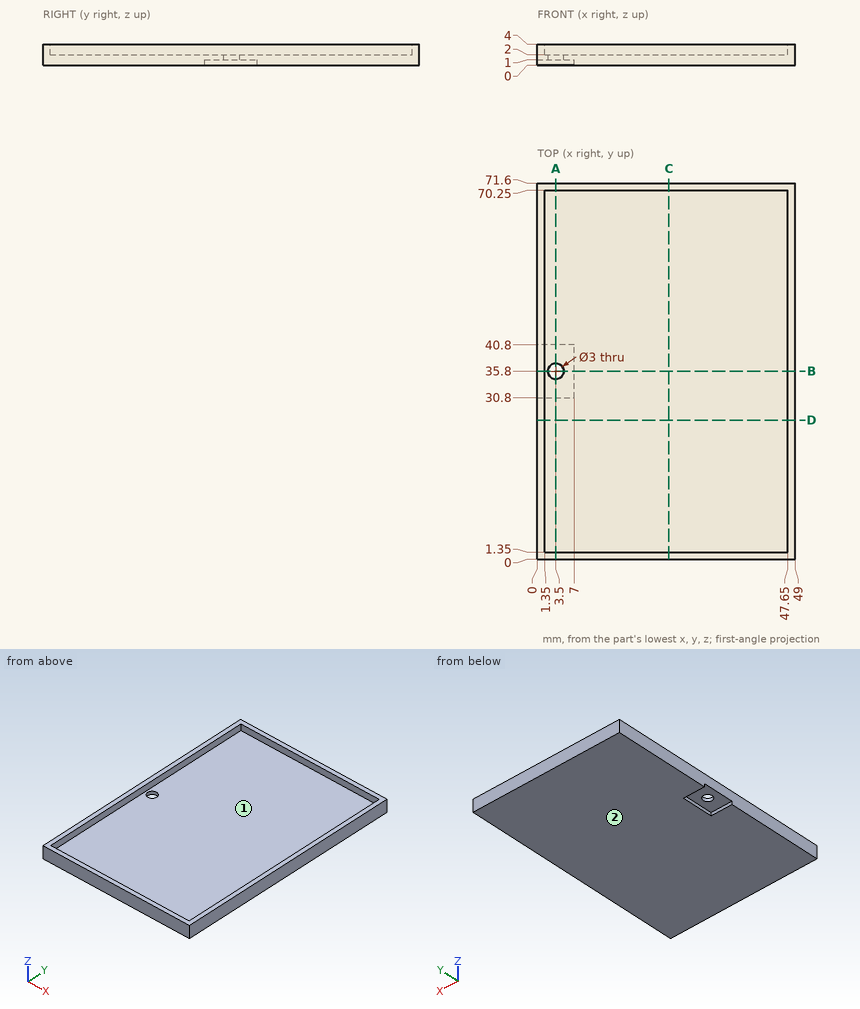
Print and shaded views of the part. All mm, measured from the part's lowest x, y and z. Round coordinates to 2 decimals unless told otherwise and drop trailing zeros. Write each loop counter-clockwise with the first axis right and the second up, starting at its lowest first coordinate (ties: lowest second). Pieces come first, ordered by that corner, then holes. Notation, with made-up numbers: M 12,4 L 52,4 A14 ccw 52,26 Z; hole C 75.25,-37.75 d3. An arc over 180 degrees is marked long. Use a Markdown table: item, result. Add a question column.
1. Slice it at A-A on x = 3.5. Give the cut face in (y, z).
2. Pull direction X, two halves, no side cores. Call the marked faces 1 and 2: released by +X, released by -X, zero draft, split by the parting line, or undercut.
3. Slice it at D-D on y = 26.5. Give the cut face in (x, z), then the cut area to 3 significant figures.
4. Flat gauge pins, fed straight in: P1, Ø4, axis at x = 26, y = 46, coming from the +Z side; P2, Ø1.1, axis at x = 4.5, z = 0.5, coming from the -Y side; P3, Ø2, axis at x = 2, y = 36, coming from the -Z side; P4, Ø0.8, axis at y = 34, z = 0.5, coming from the -X side. Where does each tip first touch, or does it go through?
5. Slice it at B-B on y = 35.8. Give the cut face in (x, z), then the cut area to 3 significant figures.
6. Slice it at C-C on x = 25. Give the cut face in (y, z).
7. Drill centre lines: probe 1 along X at (y, z) = (35.8, 1.2); probe 2 along X at (y, z) = (24.5, 2.25); probe 3 along Y at (x, z) = (10, 3.3). Where is each one in solid material? Low to high.
Reply:
| question | item | result |
|---|---|---|
| 1 | outline | M 0,0 L 30.8,0 L 30.8,1 L 34.3,1 L 34.3,2 L 1.35,2 L 1.35,4 L 0,4 Z; M 37.3,1 L 40.8,1 L 40.8,0 L 71.6,0 L 71.6,4 L 70.25,4 L 70.25,2 L 37.3,2 Z |
| 2 | face 1 | undercut |
| 2 | face 2 | zero draft |
| 3 | outline | M 0,0 L 49,0 L 49,4 L 47.65,4 L 47.65,2 L 1.35,2 L 1.35,4 L 0,4 Z |
| 3 | area | 103 mm^2 |
| 4 | P1 | stops at z = 2 |
| 4 | P2 | stops at y = 0 |
| 4 | P3 | stops at z = 1 |
| 4 | P4 | stops at x = 7 |
| 5 | outline | M 0,1 L 2,1 L 2,2 L 1.35,2 L 1.35,4 L 0,4 Z; M 5,1 L 7,1 L 7,0 L 49,0 L 49,4 L 47.65,4 L 47.65,2 L 5,2 Z |
| 5 | area | 93.4 mm^2 |
| 6 | outline | M 0,0 L 71.6,0 L 71.6,4 L 70.25,4 L 70.25,2 L 1.35,2 L 1.35,4 L 0,4 Z |
| 7 | probe 1 | x = 0 to 2, 5 to 49 |
| 7 | probe 2 | x = 0 to 1.35, 47.65 to 49 |
| 7 | probe 3 | y = 0 to 1.35, 70.25 to 71.6 |
